```python
from build123d import *

# Parameters (mm, degrees)
BOSS_EXTRUDE1_DEPTH             = 25
SKETCH2_W                       = 30
SKETCH2_H                       = 10
CUT_EXTRUDE1_DEPTH              = 107.066017178
BOSS_EXTRUDE2_REACH             = 108.066
SKETCH3_R                       = 15
SKETCH3_R_2                     = 10
BOSS_EXTRUDE2_DIRECTION_2_DEPTH = 35
CUT_EXTRUDE2_DEPTH              = 109.857705285
BOSS_EXTRUDE3_REACH             = 113.018
BOSS_EXTRUDE3_END_RADIUS        = 15
SKETCH4_W                       = 20
SKETCH4_H                       = 25
CUT_EXTRUDE3_REACH              = 113.018
CUT_EXTRUDE3_END_RADIUS         = 10
SKETCH5_R                       = 5
CUT_EXTRUDE4_REACH              = 110.858


with BuildPart() as part:
    # Sketch1 → Boss-Extrude1 (new, symmetric)
    with BuildSketch(Plane.XY):
        Polygon((0, 0), (100, 0), (100, 25), (30, 25), (30, 20), (0, 20), align=None)
    extrude(amount=BOSS_EXTRUDE1_DEPTH, both=True)

    # Sketch2 → Cut-Extrude1 (cut, through all)
    with BuildSketch(Plane.ZY):
        with Locations((0, 5)):
            Rectangle(SKETCH2_W, SKETCH2_H)
    extrude(amount=-CUT_EXTRUDE1_DEPTH, mode=Mode.SUBTRACT)

    # Boss-Extrude2: up to this face of the body (flat: up to its plane)
    boss_extrude2_end = Plane(part.part.faces().sort_by_distance((15, 20, 0))[0])
    # Sketch3 → Boss-Extrude2 (add, up to the picked face)
    with BuildSketch(Plane(origin=(0, 25, 0), x_dir=(1, 0, 0), z_dir=(0, 1, 0)), mode=Mode.PRIVATE) as boss_extrude2_sk1:
        with Locations(Location((30, 0, 0), (0, 0, 270))):
            Circle(SKETCH3_R)
        with Locations(Location((30, 0, 0), (0, 0, 90))):
            Circle(SKETCH3_R_2, mode=Mode.SUBTRACT)
    boss_extrude2_tool1 = split(extrude(boss_extrude2_sk1.sketch, amount=-BOSS_EXTRUDE2_REACH, mode=Mode.PRIVATE), bisect_by=boss_extrude2_end, keep=Keep.BOTH, mode=Mode.PRIVATE)
    add(boss_extrude2_tool1.solids().sort_by(Axis((30, 25, -14.575736), (0, -1, 0)))[0])

    # Sketch3 → Boss-Extrude2 direction 2 (add)
    with BuildSketch(Plane(origin=(0, 25, 0), x_dir=(1, 0, 0), z_dir=(0, 1, 0))):
        with Locations(Location((30, 0, 0), (0, 0, 270))):
            Circle(SKETCH3_R)
        with Locations(Location((30, 0, 0), (0, 0, 90))):
            Circle(SKETCH3_R_2, mode=Mode.SUBTRACT)
    extrude(amount=BOSS_EXTRUDE2_DIRECTION_2_DEPTH)

    # Sketch3<2> → Cut-Extrude2 (cut, through all)
    with BuildSketch(Plane(origin=(0, 25, 0), x_dir=(1, 0, 0), z_dir=(0, 1, 0))):
        with BuildLine():
            Line((30, -10), (30, 10))
            ThreePointArc((30, 10), (20, 0), (30, -10))
        make_face()
        with BuildLine():
            ThreePointArc((40, 0), (37.071067812, 7.071067812), (30, 10))
            Line((30, 10), (30, -10))
            ThreePointArc((30, -10), (37.071067812, -7.071067812), (40, 0))
        make_face()
    extrude(amount=-CUT_EXTRUDE2_DEPTH, mode=Mode.SUBTRACT)

    # Boss-Extrude3: up to this cylinder (the profile starts outside it)
    boss_extrude3_end = Plane(origin=(30, 32.5, 0), z_dir=(0, -1, 0)) * Cylinder(BOSS_EXTRUDE3_END_RADIUS, 257.036, mode=Mode.PRIVATE)
    # Sketch4 → Boss-Extrude3 (add, up to the surface)
    with BuildSketch(Plane.ZY.offset(-10), mode=Mode.PRIVATE) as boss_extrude3_sk1:
        with Locations((0, 32.5)):
            Rectangle(SKETCH4_W, SKETCH4_H)
    boss_extrude3_tool1 = extrude(boss_extrude3_sk1.sketch, amount=-BOSS_EXTRUDE3_REACH, mode=Mode.PRIVATE) - boss_extrude3_end
    add(boss_extrude3_tool1.solids().sort_by_distance((10, 32.5, 0))[0])

    # Cut-Extrude3: up to this cylinder (the profile starts outside it)
    cut_extrude3_end = Plane(origin=(30, 32.5, 0), z_dir=(0, -1, 0)) * Cylinder(CUT_EXTRUDE3_END_RADIUS, 247.036, mode=Mode.PRIVATE)
    # Sketch5 → Cut-Extrude3 (cut, up to the surface)
    with BuildSketch(Plane.ZY.offset(-10), mode=Mode.PRIVATE) as cut_extrude3_sk1:
        with Locations((0, 32.5)):
            Circle(SKETCH5_R)
    cut_extrude3_tool1 = extrude(cut_extrude3_sk1.sketch, amount=-CUT_EXTRUDE3_REACH, mode=Mode.PRIVATE) - cut_extrude3_end
    add(cut_extrude3_tool1.solids().sort_by_distance((10, 32.5, 0))[0], mode=Mode.SUBTRACT)

    # Sketch6 → Cut-Extrude4 (cut, up to next)
    with BuildSketch(Plane(origin=(0, 25, 0), x_dir=(1, 0, 0), z_dir=(0, 1, 0)), mode=Mode.PRIVATE) as cut_extrude4_sk1:
        with BuildLine():
            Line((60, 10), (85, 10))
            ThreePointArc((85, 10), (95, 0), (85, -10))
            Line((85, -10), (60, -10))
            ThreePointArc((60, -10), (50, 0), (60, 10))
        make_face()
    cut_extrude4_tool1 = extrude(cut_extrude4_sk1.sketch, amount=-CUT_EXTRUDE4_REACH, mode=Mode.PRIVATE) & part.part
    add(cut_extrude4_tool1.solids().sort_by_distance((72.5, 25, 0))[0], mode=Mode.SUBTRACT)


solid = part.part
```
Work out the finished part from the listing and answer in its coordinate system (mm). A direction names the side the tool comes from. Give positions to 0.01 mm unless a question says otherwise; leave off trailing zeros. Order: outer loops, then holes, each group sorted by start corner. A loop starts at its lowest first (then second) coordinate and runs counter-clockwise, first axis right, second up.
1. Straight lines are drawn through the part: L1, parallel to Y at x = 16.25, z = 0; L2, parallel to Y at x = 14, z = 0; L3, parallel to Z at x = 17, y = 32. For each, find the intervals that lie inside material, in ascending order.
Result sheet:
L1: y = 10 to 27.5, 37.5 to 60
L2: y = 10 to 27.5, 37.5 to 45
L3: z = -10 to -4.97, 4.97 to 10
2. Section B-B, the plane x = 77 is taken. Determine the outline of the cut face in (y, z).
Result sheet:
outline: (0, -25) - (25, -25) - (25, -10) - (10, -10) - (10, -15) - (0, -15) - close; (0, 15) - (10, 15) - (10, 10) - (25, 10) - (25, 25) - (0, 25) - close
3. Section A-A, the plane y = 6.5 is taken. Determine the outline of the cut face in (x, z).
Result sheet:
outline: (0, -25) - (100, -25) - (100, -15) - (0, -15) - close; (0, 15) - (100, 15) - (100, 25) - (0, 25) - close
4. Each of these flat-tipped pins is pushed along its axis until it touches: P1, Ø1.5, axis at y = 23.5, z = -18.5, coming from the -X side; P2, Ø16, axis at x = 30, z = 0, coming from the -Y side; P3, Ø10, axis at y = 34, z = 5.5, coming from the -X side; P4, Ø13, axis at y = 32.5, z = 0, coming from the +X side. Where does it stop, or does it pass through?
Result sheet:
P1: stops at x = 30
P2: passes through
P3: stops at x = 10
P4: stops at x = 45
5. For faces 1 (the flat face through (14, 32, -10)), 2 (the cylindrical face through (15.591, 32.72, -4.995)), 3 (the flat face through (72, 18, -10)), 4 (the flat face through (14, 32, 10)), determine the directions among +Z, -Z, +X, -X, +Y, -Y from which every point of the face is accessible in a straight line to the end or side of a thin tool.
Result sheet:
face 1: -Z, -X, +Y
face 2: -X
face 3: +Y, -Y
face 4: +Z, -X, +Y
6. Section C-C, the plane y = 22 is taken. Determine the outline of the cut face in (x, z), and give its area (3 significant figures).
Result sheet:
outline: (10, -10) - (18.82, -10) arc R15 ccw to (30, -15) - (30, -25) - (100, -25) - (100, 25) - (30, 25) - (30, 15) arc R15 ccw to (18.82, 10) - (10, 10) - close; hole circle Ø20 at (30, 0); hole (60, -10) - (85, -10) arc R10 ccw to (85, 10) - (60, 10) arc R10 ccw to start
area: 2,850 mm2
7. The mould has two halves that part along X. Classify faces 5 (the flat face through (73, 18, 10)), 6 (the flat face through (10, 35, -5)), 7 (the flat face through (100, 15, 0)), 8 (the flat face through (38, 10, -7)): released by +X, released by -X, zero draft, split by the parting line, or undercut.
Result sheet:
face 5: undercut
face 6: released by -X
face 7: released by +X
face 8: zero draft
8. Section D-D, the plane z = 2.5 is taken. Determine the outline of the cut face in (x, y), and give its area (3 significant figures).
Result sheet:
outline: (0, 10) - (20.32, 10) - (20.32, 28.17) - (10, 28.17) - (10, 20) - (0, 20) - close; (10, 36.83) - (20.32, 36.83) - (20.32, 60) - (15.21, 60) - (15.21, 45) - (10, 45) - close; (39.68, 10) - (50.32, 10) - (50.32, 25) - (44.79, 25) - (44.79, 60) - (39.68, 60) - close; (94.68, 10) - (100, 10) - (100, 25) - (94.68, 25) - close
area: 866 mm2
